Work out the finished part from the listing and answer in its coordinate system (mm). Face numbers are marked on the shaded views. A direction names the side the tool comes from. Round coordinates to 2 decimals unless told otherwise and drop trailing zeros. Loops run counter-clockwise (first coordinate to the right, second up) from the corner with the lowest first, then second, coordinate; pieces in that order, holes last. Notation, with made-up numbers: (79.5, -28) - (138.5, -28) arc R11 ccw to (138.5, -15) - close; hole circle Ø4 at (42, 5.25). An arc over 180 degrees is marked (long way). Answer as CSV lines item,"result". Start each with the question number.
Q1. Straight lines are drawn through the part: L1, parallel to Z at x = 0, y = 8; L2, parallel to Z at x = 0, y = 16; L3, parallel to X at y = 5.75, z = 6.5. For each, find the intervals that lie inside material, in ascending order. Write a range as [from, to].
Q2. For the marked faces 4, 5, 6 and 7, determine the directions among +Z, -Z, +X, -X, +Y, -Y from which every point of the face is accessible in a straight line to the end or side of a thin tool.
Q3. Section A-A on x = 0 is taken. Count the separate pieces of the cut face and the enclosed holes in it, then the cut area to 3 significant figures.
Q4. Each of these flat-tipped pins is pushed along its axis until it touches: pin 1 Ø2.5 at (x, z) = (-1.5, 6) entering from -Y; pin 2 Ø3 at (x, y) = (10.5, 7) entering from -Z; pin 3 Ø1 at (y, z) = (17.5, 6) entering from +X. Where does it stop, or does it pass through?
Q5. The mould has two halves that part along Z. Classify the marked faces 1, 2 and 3: +Z half, -Z half, draft (parallel to the pull), parting line (faces both ways), or undercut.
Q6. Section B-B on y = 10.25 is taken. Write down the section's boundary in (x, z) (3 decimals).
Q7. Section C-C on z = 31 is taken. Write down the section's boundary in (x, y).
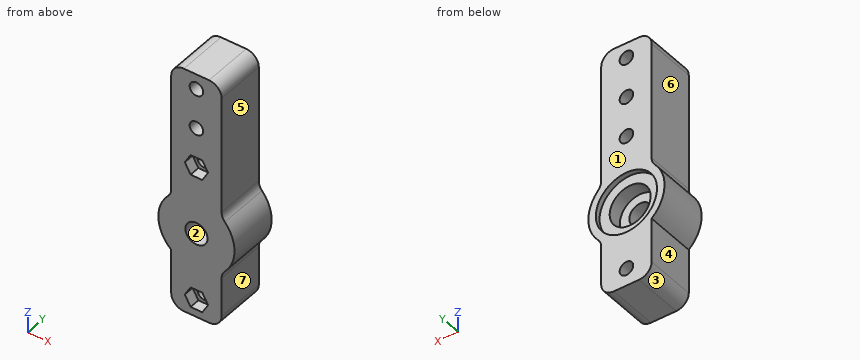
Autodesk Inventor part; units mm, degrees
ref_plane "YZ Plane" through (0, 0, 0) normal (1, 0, 0) x (0, 1, 0)
ref_plane "XZ Plane" through (0, 0, 0) normal (0, 1, 0) x (-1, 0, 0)
ref_plane "XY Plane" through (0, 0, 0) normal (0, 0, 1) x (1, 0, 0)
sketch "Boceto1" plane through (0, 0, 0) normal (0, 1, 0) x (-1, 0, 0)
  line L0 (-10, 44.5408) -> (10, 44.5408)
  line L1 (10, 44.5408) -> (10, -27.9592)
  line L2 (10, -27.9592) -> (-10, -27.9592)
  line L3 (-10, -27.9592) -> (-10, 44.5408)
  line L4 (-10, 44.5408) -> (10, -27.9592) construction
  line L5 (10, 44.5408) -> (-10, -27.9592) construction
  circle A0 centre (0, -20.4592) radius 4.4
  point P0 (0, 8.2908)
  dimension "d1" = 20
  dimension "d2" = 8.8
  dimension "d3" = 7.5
  dimension "d26" = 65
extrude "Extrusión1" add sketch "Boceto1" along normal blind 20
sketch "Boceto2" plane through (0, 20, 0) normal (0, 1, 0) x (1, 0, 0)
  circle A0 centre (0, 20.4592) radius 4.4
  circle A1 centre (0, 20.4592) radius 12.125
  point P0 (0, 0)
  dimension "d6" = 24.25
extrude "Extrusión2" cut sketch "Boceto2" against normal blind 2.5
sketch "Boceto3" plane through (0, 20, 0) normal (0, 1, 0) x (1, 0, 0)
  circle A0 centre (0, 20.4592) radius 4.4
  circle A1 centre (0, 20.4592) radius 12.125
  circle A2 centre (0, 20.4592) radius 15.125
  line L0 (10, 27.316) -> (10, 13.6024)
  arc A3 (10, 27.316) -> (9.5271, 27.9592) centre (0, 20.4592) ccw
  line L1 (-9.5271, 27.9592) -> (9.5271, 27.9592)
  arc A4 (-9.5271, 27.9592) -> (-10, 27.316) centre (0, 20.4592) ccw
  line L2 (-10, 13.6024) -> (-10, 27.316)
  arc A5 (-10, 13.6024) -> (10, 13.6024) centre (0, 20.4592) ccw
  circle A6 centre (0, 20.4592) radius 4.4
  point P0 (0, 0)
  point P1 (-10, 27.316)
  point P2 (10, 27.316)
  point P3 (9.5271, 27.9592)
  dimension "d9" = 3
extrude "Extrusión3" add sketch "Boceto3" against normal up to surface (20 mm away) contours A1 L0 | L1 A1 | A1 L2 | A2
sketch "Boceto4" plane through (0, 20, 0) normal (0, 1, 0) x (1, 0, 0)
  circle A0 centre (0, 20.4592) radius 4.4
  circle A1 centre (0, 20.4592) radius 12.15
  point P0 (0, 0)
  dimension "d14" = 24.3
extrude "Extrusión4" cut sketch "Boceto4" against normal blind 2 contours A0 | A1
sketch "Boceto5" plane through (0, 17.5, 0) normal (0, 1, 0) x (1, 0, 0)
  line L0 (10, 27.316) -> (10, 13.6024)
  arc A0 (10, 27.316) -> (9.5271, 27.9592) centre (0, 20.4592) ccw
  line L1 (-9.5271, 27.9592) -> (9.5271, 27.9592)
  arc A1 (-9.5271, 27.9592) -> (-10, 27.316) centre (0, 20.4592) ccw
  line L2 (-10, 13.6024) -> (-10, 27.316)
  arc A2 (-10, 13.6024) -> (10, 13.6024) centre (0, 20.4592) ccw
  circle A3 centre (0, 20.4592) radius 4.4
  point P0 (0, 0)
extrude "Extrusión5" add sketch "Boceto5" along normal up to surface (0.5 mm away)
sketch "Boceto6" plane through (0, 0, 0) normal (0, -1, 0) x (1, 0, 0)
  circle A0 centre (0, 38.5408) radius 2.7
  circle A1 centre (0, 22.5408) radius 2.7
  line L0 (-10, 44.5408) -> (10, 44.5408)
  circle A2 centre (0, 6.5408) radius 2.7
  point P0 (0, 0)
  dimension "d20" = 16
  dimension "d21" = 5.4
  dimension "d30" = 6
  dimension "d35" = 16
extrude "Extrusión6" cut sketch "Boceto6" against normal through all
sketch "Boceto8" plane through (0, 18, -20.4592) normal (0, 1, 0) x (1, 0, 0)
  circle A0 centre (0, 0) radius 4.4
  circle A1 centre (0, 0) radius 8.125
  point P0 (0, -20.4592)
  dimension "d31" = 16.25
extrude "Extrusión8" cut sketch "Boceto8" against normal blind 5.5 contours A0 | A1
fillet "Empalme4" radius 5 4 edges at (10, 10, 44.5408) (-10, 10, 44.5408) (10, 10, -9.1117) (-10, 10, -9.1117)
sketch "Boceto9" plane through (0, 20, 0) normal (0, 1, 0) x (1, 0, 0)
  arc A0 (11.2733, 10.3756) -> (-11.2733, 10.3756) centre (0, 20.4592) ccw
  line L0 (-10, 31.8067) -> (10, 31.8067)
  line L1 (10, 31.8067) -> (10, 54.4592)
  line L2 (10, 54.4592) -> (-10, 54.4592)
  line L3 (-10, 54.4592) -> (-10, 31.8067)
  line L4 (-10, 7.0422) -> (-10, -39.5408)
  line L5 (10, -39.5408) -> (10, 7.0422)
  circle A1 centre (0, 20.4592) radius 21
  circle A2 centre (0, 47.4592) radius 2.7
  point P0 (0, 0)
  dimension "d36" = 42
  dimension "d37" = 34
  dimension "d38" = 5.4
  dimension "d39" = 7
extrude "Extrusión9" add sketch "Boceto9" against normal up to surface (20 mm away) contours A0 L3 A1 L1 | A1 L3 L2 L1
fillet "Empalme5" radius 5 3 edges at (10, 10, -31.8067) (10, 10, -54.4592) (-10, 10, -54.4592)
sketch "Boceto10" plane through (0, 0, 0) normal (0, -1, 0) x (1, 0, 0)
  circle A0 centre (0, -47.4592) radius 2.7
  circle A1 centre (0, -47.4592) radius 4
  circle A2 centre (0, 6.5408) radius 2.7
  circle A3 centre (0, 6.5408) radius 4
  line L0 (-4.6188, -47.4592) -> (-2.3094, -43.4592)
  line L1 (-2.3094, -43.4592) -> (2.3094, -43.4592)
  line L2 (2.3094, -43.4592) -> (4.6188, -47.4592)
  line L3 (4.6188, -47.4592) -> (2.3094, -51.4592)
  line L4 (2.3094, -51.4592) -> (-2.3094, -51.4592)
  line L5 (-2.3094, -51.4592) -> (-4.6188, -47.4592)
  line L6 (-4.6188, 6.5408) -> (-2.3094, 10.5408)
  line L7 (-2.3094, 10.5408) -> (2.3094, 10.5408)
  line L8 (2.3094, 10.5408) -> (4.6188, 6.5408)
  line L9 (4.6188, 6.5408) -> (2.3094, 2.5408)
  line L10 (2.3094, 2.5408) -> (-2.3094, 2.5408)
  line L11 (-2.3094, 2.5408) -> (-4.6188, 6.5408)
  point P0 (0, 0)
  dimension "d43" = 8
extrude "Extrusión10" cut sketch "Boceto10" against normal blind 4.2 contours A0 | A1 | A1 L2 L3 | A1 L1 L2 | L3 L4 A1 | A1 L0 L1 | L4 L5 A1 | A1 L5 L0 | A2 | A3 | A3 L8 L9 | A3 L7 L8 | L9 L10 A3 | A3 L6 L7 | L10 L11 A3 | A3 L11 L6
sketch "Boceto7" plane through (0, 0, 0) normal (0, -1, 0) x (1, 0, 0)
  circle A0 centre (0, -20.4592) radius 2.65
  circle A1 centre (0, -20.4592) radius 4.05
  line L0 (0, -25.1357) -> (-4.05, -22.7975)
  line L1 (-4.05, -22.7975) -> (-4.05, -18.1209)
  line L2 (-4.05, -18.1209) -> (0, -15.7826)
  line L3 (0, -15.7826) -> (4.05, -18.1209)
  line L4 (4.05, -18.1209) -> (4.05, -22.7975)
  line L5 (4.05, -22.7975) -> (0, -25.1357)
  point P0 (0, 0)
  dimension "d27" = 8.1
properties part number "bottomsupport"
Findings:
1,L1,"z = [-54.46, -50.16], [-44.76, -24.86], [-16.06, 3.84], [9.24, 19.84], [25.24, 35.84], [41.24, 44.54]"
1,L2,"z = [-54.46, -50.16], [-44.76, -28.58], [-12.33, 3.84], [9.24, 19.84], [25.24, 35.84], [41.24, 44.54]"
1,L3,"x = [-10, -2.7], [2.7, 10]"
2,face 4,"-Z, -X, +Y, -Y"
2,face 5,"+Z, +X, +Y, -Y"
2,face 6,"+Z, -X, +Y, -Y"
2,face 7,"-Z, +X, +Y, -Y"
3,separate pieces,"6"
3,enclosed holes,"0"
3,area,"1,280 mm^2"
4,pin 1,"stops at y = 4.2"
4,pin 2,"stops at z = -52.46"
4,pin 3,"stops at x = 10"
5,face 1,"draft"
5,face 2,"undercut"
5,face 3,"-Z half"
6,outline,"(-11.273, -10.376) arc R15.125 ccw to (-10, -31.807) - (-10, -49.459) arc R5 ccw to (-5, -54.459) - (5, -54.459) arc R5 ccw to (10, -49.459) - (10, -33.876) arc R5 cw to (11.273, -30.543) arc R15.125 ccw to (11.273, -10.376) arc R5 cw to (10, -7.042) - (10, 39.541) arc R5 ccw to (5, 44.541) - (-5, 44.541) arc R5 ccw to (-10, 39.541) - (-10, -7.042) arc R5 cw to start; hole circle Ø8.8 at (0, -20.459); hole circle Ø5.4 at (0, -47.459); hole circle Ø5.4 at (0, 6.541); hole circle Ø5.4 at (0, 22.541); hole circle Ø5.4 at (0, 38.541)"
7,outline,"(-10, 0) - (10, 0) - (10, 20) - (-10, 20) - close"
